The listing builds one solid part. Answer for the finished solid, in the listing's coordinates (mm). Face numbers are marked on the shaded views. Round coordinates to 2 decimals unless told otherwise and drop trailing zeros. Loops run counter-clockwise (first coordinate to the right, second up) from the corner with the lowest first, then second, coordinate; pieces in that order, holes last. Notation, with made-up numbers: (34.25, 3) - (38.25, 3) arc R31 cw to (38.25, 42) - close; hole circle Ø3 at (7.25, -16.5). An arc over 180 degrees is marked (long way). One line per question, with ' | ' between items. Start each with the question number.
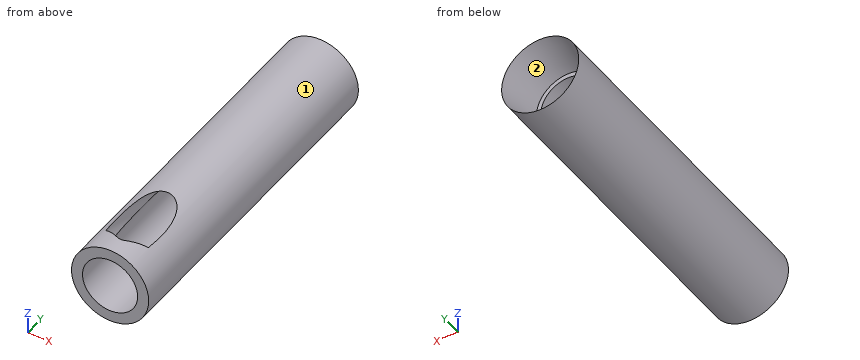
from build123d import *

# Parameters (mm, degrees)
F5_D     = 20
F5_DEPTH = 50
F5_TIP   = 6.0086061903


with BuildPart() as f1:
    # F0 (on Top) → F1 (revolve)
    with BuildSketch(Plane.XY):
        Polygon((12.5, 129.8480927944), (12.5, 0), (17.5, 0), (17.5, 60), (17.5, 150), (14.5, 129.8480927944), align=None)
    revolve(axis=Axis((0, 75, 0), (0, 1, 0)))

    # F5 (one way)
    with BuildSketch(Plane(origin=(0, 52.9813332936, -19.2836282906), x_dir=(-1, 0, 0), z_dir=(0, 0.9396926208, -0.3420201433))):
        with Locations((0, 20.5212085995)):
            Circle(F5_D / 2)
    extrude(amount=-F5_DEPTH, mode=Mode.SUBTRACT)
    with Locations(Plane(origin=(0, 52.9813332936, -19.2836282906), x_dir=(-1, 0, 0), z_dir=(0, 0.9396926208, -0.3420201433))):
        with Locations((0, 20.5212085995)):
            with Locations((0, 0, -(F5_DEPTH + F5_TIP / 2))):  # 118° drill point
                Cone(0, F5_D / 2, F5_TIP, mode=Mode.SUBTRACT)


solid = f1.part
(1) Find section B-B on x = 0. Write down the section's boundary in (y, z), plus the area to 3 significant figures.
(2) Determine the mould class of the marked faces 1 and 2 for opening direction Z: pulls with the +Z half, pulls with the -Z half, needs draft (parallel to the pull), parting line crosses it, or undercut.
(3) Find section A-A on z = 0. Write down the section's boundary in (x, y), plus the area to 3 significant figures.
(4) Each of these flat-tipped pins is pushed along its axis until it touches: P1, Ø2, axis at y = 127.5, z = 2.5, coming from the +X side; P2, Ø1.5, axis at x = 13.5, y = 97, coming from the -Z side; P3, Ø5, axis at y = 47, z = -11, coming from the -X side; P4, Ø4, axis at x = 3.5, z = 13, coming from the -Y side. Where does it stop, or does it pass through?
(5) Consider L1, parallel to X at y = 84, z = 0; L2, parallel to X at y = 74.5, z = 7; L3, parallel to Z at x = 0, y = 34. Determine where each line is inside the solid, lowest interval first.
(6) Find section C-C on y = 112. Write down the section's boundary in (x, z), plus the area to 3 significant figures.
Answer below:
1) outline: (0, -17.5) - (150, -17.5) - (129.85, -14.5) - (129.85, -12.5) - (0, -12.5) - close; (0, 12.5) - (8.66, 12.5) - (7.69, 17.5) - (0, 17.5) - close; (41.16, 17.5) - (54.89, 12.5) - (129.85, 12.5) - (129.85, 14.5) - (150, 17.5) - close | area: 1,160 mm2
2) face 1: parting line crosses it | face 2: undercut
3) outline: (-17.5, 0) - (-12.5, 0) - (-12.5, 129.85) - (-14.5, 129.85) - (-17.5, 150) - close; (12.5, 0) - (17.5, 0) - (17.5, 150) - (14.5, 129.85) - (12.5, 129.85) - close | area: 1,360 mm2
4) P1: x = 17.44 | P2: z = -11.99 | P3: x = -15.3 | P4: y = 0
5) L1: -17.5 to -12.5, 12.5 to 17.5 | L2: -16.04 to -10.36, 10.36 to 16.04 | L3: -17.5 to -12.5
6) outline: circle Ø35 at (0, 0); hole circle Ø25 at (0, 0) | area: 471 mm2
